```python
from build123d import *

# Parameters (mm, degrees)
SKETCH1_R           = 13
BOSS_EXTRUDE1_DEPTH = 2
SKETCH2_R           = 1.5
CUT_EXTRUDE1_DEPTH  = 19.493242009
BOSS_EXTRUDE2_DEPTH = 50
CHAMFER1_SIZE       = 5


with BuildPart() as part:
    # Sketch1 → Boss-Extrude1 (new body)
    with BuildSketch(Plane(origin=(0, 0, 0), x_dir=(1, 0, 0), z_dir=(0, 1, 0))):
        with Locations(Location((0, 0, 0), (0, 0, 270))):
            Circle(SKETCH1_R)
    extrude(amount=BOSS_EXTRUDE1_DEPTH)

    # Sketch2 → Cut-Extrude1 (cut, through all)
    with BuildSketch(Plane(origin=(0, 2, 0), x_dir=(1, 0, 0), z_dir=(0, 1, 0))):
        with Locations(Location((-8, 0, 0), (0, 0, 270))):
            Circle(SKETCH2_R)
        with Locations(Location((0, 8, 0), (0, 0, 270))):
            Circle(SKETCH2_R)
        with Locations(Location((8, 0, 0), (0, 0, 270))):
            Circle(SKETCH2_R)
        with Locations(Location((0, -8, 0), (0, 0, 270))):
            Circle(SKETCH2_R)
    extrude(amount=-CUT_EXTRUDE1_DEPTH, mode=Mode.SUBTRACT)

    # Sketch3 → Boss-Extrude2 (add)
    with BuildSketch(Plane(origin=(0, 2, 0), x_dir=(1, 0, 0), z_dir=(0, 1, 0))):
        with BuildLine():
            ThreePointArc((-7.6687375, 10.497164625), (-9.192388155, 9.192388155), (-10.497164625, 7.6687375))
            Line((-10.497164625, 7.6687375), (-2.828427125, 0))
            Line((-2.828427125, 0), (-10.497164625, -7.6687375))
            ThreePointArc((-10.497164625, -7.6687375), (-9.192388155, -9.192388155), (-7.6687375, -10.497164625))
            Line((-7.6687375, -10.497164625), (0, -2.828427125))
            Line((0, -2.828427125), (7.6687375, -10.497164625))
            ThreePointArc((7.6687375, -10.497164625), (9.192388155, -9.192388155), (10.497164625, -7.6687375))
            Line((10.497164625, -7.6687375), (2.828427125, 0))
            Line((2.828427125, 0), (10.497164625, 7.6687375))
            ThreePointArc((10.497164625, 7.6687375), (9.192388155, 9.192388155), (7.6687375, 10.497164625))
            Line((7.6687375, 10.497164625), (0, 2.828427125))
            Line((0, 2.828427125), (-7.6687375, 10.497164625))
        make_face()
    extrude(amount=BOSS_EXTRUDE2_DEPTH)

    # Chamfer1
    chamfer1_edges = [part.edges().sort_by_distance(p)[0] for p in [
        (-9.192388155, 52, 9.192388155),
        (9.192388155, 52, 9.192388155),
        (9.192388155, 52, -9.192388155),
        (-9.192388155, 52, -9.192388155),
    ]]
    chamfer(chamfer1_edges, length=CHAMFER1_SIZE)


solid = part.part
```
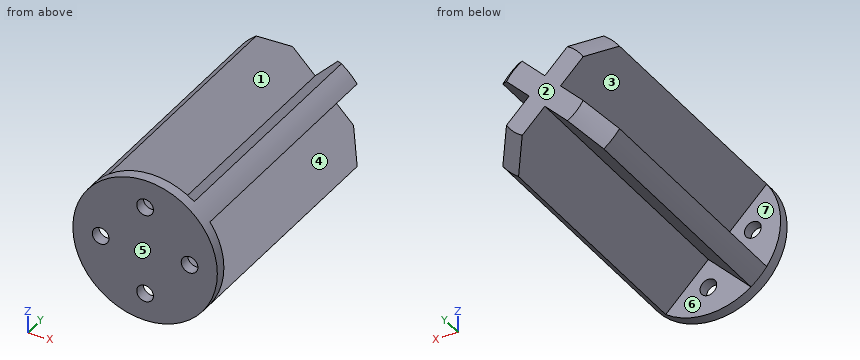
Design review of the part built by this model. Coordinates are the model's own, in mm. Face numbers are marked on the shaded views. A direction names the side the tool comes from. Coordinates: 2 decimals unless noted, no trailing zeros. Order: outer loops, then holes, each group sorted by start corner. A loop starts at its lowest first (then second) coordinate and runs counter-clockwise, first axis right, second up. Notation, with made-up numbers: (59, 82) -> (77, 82) arc R18 cw to (77, 104) -> close; hole circle Ø7 at (62, 51). An arc over 180 degrees is marked (long way). One line per item, written item: value. Start each with the question number.
Q1. Take a section at A-A, the plane x = 0.75. State the section outline as (y, z) points, then the cut area to 3 significant figures.
Q2. Mouldability with a two-part tool opening along X and no side actions: class the marked faces 1, 2 and 3 as pulls with the +X half, pulls with the -X half, needs draft (parallel to the pull), parting line crosses it, or undercut.
Q3. For probe 1 along X at (y, z) = (1.5, 0); probe 2 along Y at (x, z) = (-6, 0.25); probe 3 along X at (y, z) = (40, -7.75), list the stretches that pass through material, from the lowest coordinate up.
Q4. Tool access review of the marked faces 4, 5, 6 and 7: name each direction out of +Z, -Z, +X, -X, +Y, -Y from which nothing blocks a thin tool from reaching the whole face with its end or side.
Q5. Insertion check: pin 1 Ø3 at (x, y) = (-9, 31) entering from -Z; pin 2 Ø5 at (x, z) = (8.5, -2) entering from +Y; pin 3 Ø3 at (x, y) = (2, 30.5) entering from +Z; pin 4 Ø2.5 at (x, z) = (8, 0) entering from +Y (1 decimal). Each pin has a flat end and moves straight along its axis. Give the tip position at first contact, or say it passes through.
Q6. Take a section at B-B, the plane y = 6.5. State the section outline as (x, z) points, then the cut area to 3 significant figures.
Values follow:
1. outline: (0, -12.98) -> (2, -12.98) -> (2, -9.3) -> (0, -9.3) -> close; (0, -6.7) -> (2, -6.7) -> (2, -3.58) -> (52, -3.58) -> (52, 3.58) -> (2, 3.58) -> (2, 6.7) -> (0, 6.7) -> close; (0, 9.3) -> (2, 9.3) -> (2, 12.98) -> (0, 12.98) -> close
1. area: 399 mm2
2. face 1: undercut
2. face 2: needs draft
2. face 3: pulls with the -X half
3. probe 1: x = -13 to -9.5, -6.5 to 6.5, 9.5 to 13
3. probe 2: y = 0 to 2
3. probe 3: x = -10.44 to -4.92, 4.92 to 10.44
4. face 4: +X, +Y
4. face 5: +Z, -Z, +X, -X, -Y
4. face 6: -Z, +Y
4. face 7: -X, +Y
5. pin 1: stops at z = -10.5
5. pin 2: stops at y = 2
5. pin 3: stops at z = 6.33
5. pin 4: passes through
6. outline: (-10.5, -7.67) arc R13 ccw to (-7.67, -10.5) -> (0, -2.83) -> (7.67, -10.5) arc R13 ccw to (10.5, -7.67) -> (2.83, 0) -> (10.5, 7.67) arc R13 ccw to (7.67, 10.5) -> (0, 2.83) -> (-7.67, 10.5) arc R13 ccw to (-10.5, 7.67) -> (-2.83, 0) -> close
6. area: 191 mm2
